Check sheet for the modelled part. Datum: model origin and axes. Units: mm. A direction names the side the tool comes from. Round coordinates to 2 decimals unless told otherwise and drop trailing zeros. Order: outer loops, then holes, each group sorted by start corner. A loop starts at its lowest first (then second) coordinate and runs counter-clockwise, first axis right, second up.
from build123d import *

# Parameters (mm, degrees)
SKETCH_1_R      = 1.65
SKETCH_1_R_2    = 13
EXTRUDE_1_DEPTH = 15


with BuildPart() as part:
    # 草图1 → 凸台-拉伸1 (new body)
    with BuildSketch(Plane.XY):
        with BuildLine():
            Line((-85.245113537, 20.900392521), (-339.479111624, 25.994781694))
            ThreePointArc((-339.479111624, 25.994781694), (-366, 0), (-339.479111624, -25.994781694))
            Line((-339.479111624, -25.994781694), (-85.245113537, -20.900392521))
            ThreePointArc((-85.245113537, -20.900392521), (-53.416829007, -24.942544633), (-24.108780491, -37.996930182))
            ThreePointArc((-24.108780491, -37.996930182), (45, 0), (-24.108780491, 37.996930182))
            ThreePointArc((-24.108780491, 37.996930182), (-53.416829007, 24.942544633), (-85.245113537, 20.900392521))
        make_face()
        with Locations((0, 40)):
            Circle(SKETCH_1_R, mode=Mode.SUBTRACT)
        with Locations((34.641016151, 20)):
            Circle(SKETCH_1_R, mode=Mode.SUBTRACT)
        with Locations((34.641016151, -20)):
            Circle(SKETCH_1_R, mode=Mode.SUBTRACT)
        with Locations((0, -40)):
            Circle(SKETCH_1_R, mode=Mode.SUBTRACT)
        with Locations((-34.641016151, 20)):
            Circle(SKETCH_1_R, mode=Mode.SUBTRACT)
        with Locations((-34.641016151, -20)):
            Circle(SKETCH_1_R, mode=Mode.SUBTRACT)
        with Locations((-340, 0)):
            Circle(SKETCH_1_R_2, mode=Mode.SUBTRACT)
        with BuildLine():
            Line((-35.500051413, 6.790401018), (-36.237951224, 6.373427606))
            ThreePointArc((-36.237951224, 6.373427606), (-36.795555255, 5.823507629), (-37, 5.067507244))
            Line((-37, 5.067507244), (-37, -5.067507244))
            ThreePointArc((-37, -5.067507244), (-36.795555255, -5.823507629), (-36.237951224, -6.373427606))
            Line((-36.237951224, -6.373427606), (-35.500051413, -6.790401018))
            ThreePointArc((-35.500051413, -6.790401018), (-34.451431588, -7.698788042), (-33.838125094, -8.943225935))
            ThreePointArc((-33.838125094, -8.943225935), (35, 0), (-33.838125094, 8.943225935))
            ThreePointArc((-33.838125094, 8.943225935), (-34.451431588, 7.698788042), (-35.500051413, 6.790401018))
        make_face(mode=Mode.SUBTRACT)
    extrude(amount=EXTRUDE_1_DEPTH)


solid = part.part
1) Sectioned sample at D-D on y = -30. Record the cut outline in (x, z).
2) Sectioned sample at A-A on y = 0. Record the cut outline in (x, z), and give its area (4 significant figures).
3) Gauge pin test, flat ends, axial feed: pin 1 (4 mm diameter, centred on y = 19.5, z = 6.5, fed in from +X); pin 2 (8 mm diameter, centred on x = -268.5, y = -25, fed in from +Z); pin 3 (2.5 mm diameter, centred on x = 0, y = 40, fed in from -Z); pin 4 (1.5 mm diameter, centred on x = -91, z = 12.5, fed in from -Y). Record the tip position at first contact, or that the pin passes through.
4) Set-up check for faces 1 (the face through (-163, 1, 15)), 2 (the face through (-52.983, 25.065, 7.395)), 3 (the face through (-37, 0, 7)): record each of +Z, -Z, +X, -X, +Y, -Y from which the full face is reachable in a straight line by a thin tool's end or side.
5) Sectioned sample at B-B on z = 7.75. Count the separate pieces of the cut face and the enclosed holes in it, and give its area (3 significant figures).
6) Sectioned sample at C-C on x = -330.5. Record the cut outline in (y, z).
7) Draft check along X on faces 4 (the face through (44.98, -1.35, 7.4)), 5 (the face through (-163, 1, 0)), 6 (the face through (-53.851, -24.822, 7.395)). Enter one of: pulls with the +X half, pulls with the -X half, needs draft (parallel to the pull), parting line crosses it, or undercut.
8) Scan lines: line 1 (X direction, y = -0.5, z = 13.25); line 2 (Y direction, x = 0, z = 3); line 3 (X direction, y = -19.5, z = 1). Record each from-to range of solid material in increasing order.
Values found:
1. outline: (-39.18, 0) - (-18.03, 0) - (-18.03, 15) - (-39.18, 15) - close; (18.03, 0) - (33.54, 0) - (33.54, 15) - (18.03, 15) - close
2. outline: (-366, 0) - (-353, 0) - (-353, 15) - (-366, 15) - close; (-327, 0) - (-37, 0) - (-37, 15) - (-327, 15) - close; (35, 0) - (45, 0) - (45, 15) - (35, 15) - close
2. area: 4,695 mm2
3. pin 1: stops at x = 41.46
3. pin 2: stops at z = 15
3. pin 3: passes through
3. pin 4: stops at y = -21.03
4. face 1: +Z, +X, -X, +Y, -Y
4. face 2: +Z, -Z, +Y
4. face 3: +Z, -Z
5. separate pieces: 1
5. enclosed holes: 8
5. area: 17,000 mm2
6. outline: (-25.81, 0) - (-8.87, 0) - (-8.87, 15) - (-25.81, 15) - close; (8.87, 0) - (25.81, 0) - (25.81, 15) - (8.87, 15) - close
7. face 4: parting line crosses it
7. face 5: needs draft
7. face 6: undercut
8. line 1: x = -366 to -352.99, -327.01 to -37, 35 to 45
8. line 2: y = -45 to -41.65, -38.35 to -35, 35 to 38.35, 41.65 to 45
8. line 3: x = -357.2 to -36.21, -33.07 to -29.06, 29.06 to 33.07, 36.21 to 40.56
